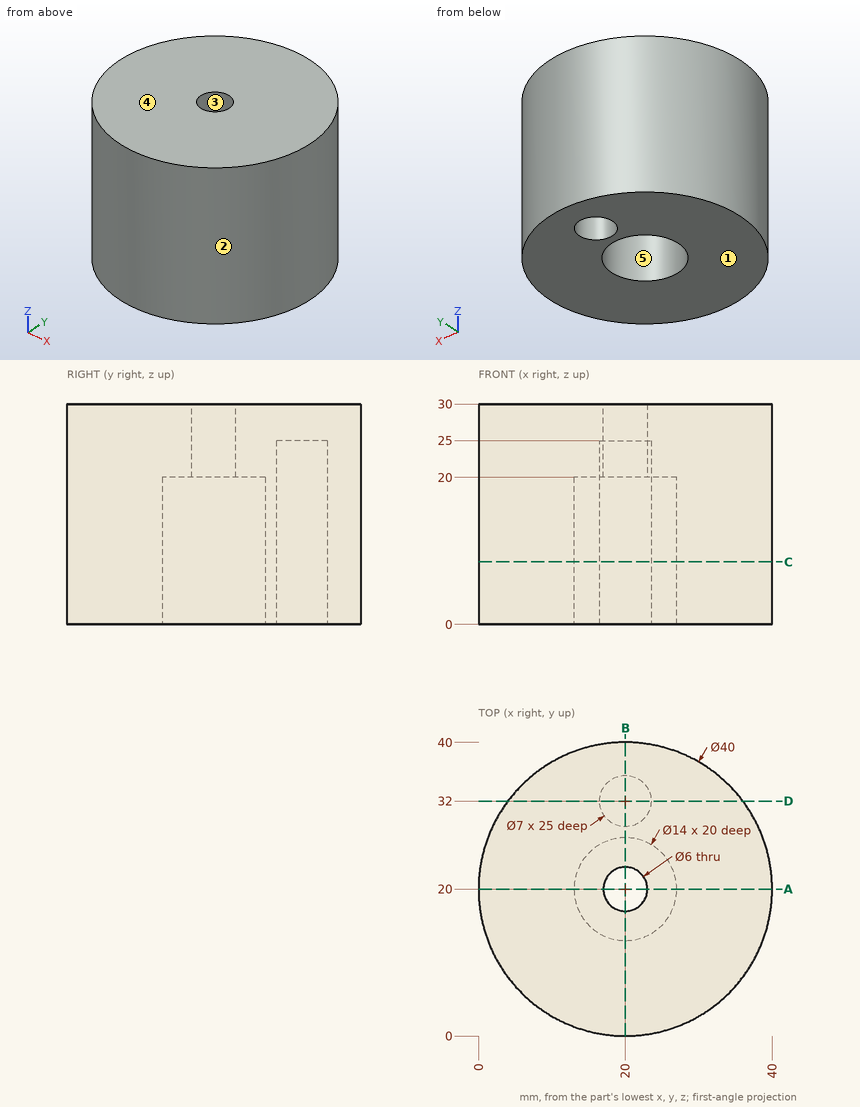
Here's the drawing with two shaded views (mm, measured from the low corner). I have some questions. A direction names the side the tool comes from. Coordinates: 2 decimals unless noted, no trailing zeros. Order: outer loops, then holes, each group sorted by start corner. A loop starts at its lowest first (then second) coordinate and runs counter-clockwise, first axis right, second up.
Item 1: For the marked faces 4 and 5, which set-ups out of +Z, -Z, +X, -X, +Y, -Y let a thin tool reach every point of the face, with its end or its side?
Result sheet:
face 4: +Z, +X, -X, +Y, -Y
face 5: -Z
Item 2: For P1, Ø5, axis at x = 20, y = 20, coming from the -Z side; P2, Ø6, axis at x = 19, z = 15.5, coming from the +Y side; P3, Ø10, axis at y = 7.5, z = 13, coming from the +X side; P4, Ø7.5, axis at x = 21.5, y = 31.5, coming from the -Z side, each with a flat end and sliding along its axis, tell me the tip position at first contact or that it passes through.
Result sheet:
P1: passes through
P2: stops at y = 40
P3: stops at x = 38.54
P4: stops at z = 0
Item 3: If we mould it in two halves opening along X, with no side actions, what happens to the marked faces 1, 2 and 3? For each: +X half, -X half, draft (parallel to the pull), parting line (faces both ways), or undercut.
Result sheet:
face 1: draft
face 2: parting line
face 3: undercut
Item 4: If we section it at B-B on x = 20: List the corners of the cut face in (y, z) for me.
Result sheet:
outline: (0, 0) - (13, 0) - (13, 20) - (17, 20) - (17, 30) - (0, 30) - close; (23, 20) - (27, 20) - (27, 0) - (28.5, 0) - (28.5, 25) - (35.5, 25) - (35.5, 0) - (40, 0) - (40, 30) - (23, 30) - close
Item 5: If we section it at A-A on y = 20: List the corners of the cut face in (x, z) for me.
Result sheet:
outline: (0, 0) - (13, 0) - (13, 20) - (17, 20) - (17, 30) - (0, 30) - close; (23, 20) - (27, 20) - (27, 0) - (40, 0) - (40, 30) - (23, 30) - close
Item 6: If we section it at C-C on z = 8.5: List the corners of the cut face in (x, y) for me.
Result sheet:
outline: circle Ø40 at (20, 20); hole circle Ø14 at (20, 20); hole circle Ø7 at (20, 32)
Item 7: I need wall thicknesses on line 1 (Y direction, x = 20, z = 5); line 2 (Y direction, x = 20, z = 22); line 3 (Y direction, x = 20, z = 26.25). Which ranges of each line are inside material? Lowest first, please.
Result sheet:
line 1: y = 0 to 13, 27 to 28.5, 35.5 to 40
line 2: y = 0 to 17, 23 to 28.5, 35.5 to 40
line 3: y = 0 to 17, 23 to 40
Item 8: If we section it at D-D on y = 32: List the corners of the cut face in (x, z) for me, plus the area to 3 significant figures.
Result sheet:
outline: (4, 0) - (16.5, 0) - (16.5, 25) - (23.5, 25) - (23.5, 0) - (36, 0) - (36, 30) - (4, 30) - close
area: 785 mm2
